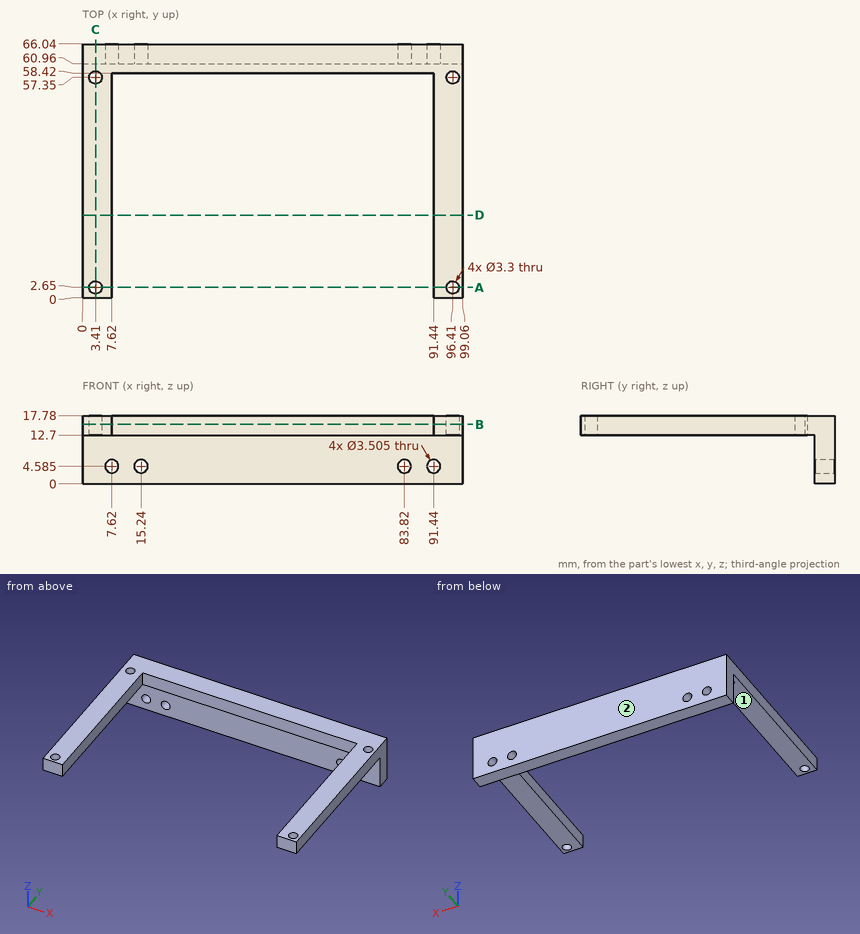
Part print with two shaded views. Sizes in mm from the minimum x, y, z corner. A direction names the side the tool comes from. Round coordinates to 2 decimals unless told otherwise and drop trailing zeros. Write each loop counter-clockwise with the first axis right and the second up, starting at its lowest first coordinate (ties: lowest second). Pieces come first, ordered by that corner, then holes. Notation, with made-up numbers: (38.5, -26) - (94.5, -26) arc R14 cw to (94.5, -22) - close; hole circle Ø7 at (65, 81). An arc over 180 degrees is marked (long way). Use CSV: the item, a comma, the result in double quotes.
Item 1: Slice it at D-D, the plane y = 21.5. Write the cut outline in (x, z), then the cut area to 3 significant figures.
Results list:
outline,"(0, 12.7) - (7.62, 12.7) - (7.62, 17.78) - (0, 17.78) - close; (91.44, 12.7) - (99.06, 12.7) - (99.06, 17.78) - (91.44, 17.78) - close"
area,"77.4 mm²"
Item 2: Flat gauge pins, fed straight in: P1, Ø2.5, axis at x = 3.41, y = 57.35, coming from the +Z side; P2, Ø1.5, axis at x = 43, z = 15, coming from the -Y side; P3, Ø6.5, axis at x = 47, z = 6.5, coming from the -Y side. Where does each tip first touch, or does it go through?
Results list:
P1,"passes through"
P2,"stops at y = 58.42"
P3,"stops at y = 60.96"
Item 3: Slice it at B-B, the plane z = 15.5. Write the cut outline in (x, y).
Results list:
outline,"(0, 0) - (7.62, 0) - (7.62, 58.42) - (91.44, 58.42) - (91.44, 0) - (99.06, 0) - (99.06, 66.04) - (0, 66.04) - close; hole circle Ø3.3 at (3.41, 2.65); hole circle Ø3.3 at (3.41, 57.35); hole circle Ø3.3 at (96.41, 2.65); hole circle Ø3.3 at (96.41, 57.35)"
Item 4: Wall check: L1, parallel to X at y = 23, z = 15; L2, parallel to Y at x = 36, z = 12; L3, parallel to Z at x = 91.44, y = 62.65. Give the ranges that are in metal, low to high.
Results list:
L1,"x = 0 to 7.62, 91.44 to 99.06"
L2,"y = 60.96 to 66.04"
L3,"z = 0 to 2.83, 6.34 to 17.78"
Item 5: Tool access for the marked faces 1 and 2: list every direction of +Z, -Z, +X, -X, +Y, -Y with a clear straight run to the whole face (end or side of a thin tool).
Results list:
face 1,"-Z, +X, -X, -Y"
face 2,"+Z, -Z, +X, -X, +Y"
Item 6: Slice it at C-C, the plane x = 3.41. Write the cut outline in (y, z).
Results list:
outline,"(0, 12.7) - (1, 12.7) - (1, 17.78) - (0, 17.78) - close; (4.3, 12.7) - (55.7, 12.7) - (55.7, 17.78) - (4.3, 17.78) - close; (59, 12.7) - (60.96, 12.7) - (60.96, 0) - (66.04, 0) - (66.04, 17.78) - (59, 17.78) - close"
Item 7: Slice it at A-A, the plane y = 2.65. Write the cut outline in (x, z).
Results list:
outline,"(0, 12.7) - (1.76, 12.7) - (1.76, 17.78) - (0, 17.78) - close; (5.06, 12.7) - (7.62, 12.7) - (7.62, 17.78) - (5.06, 17.78) - close; (91.44, 12.7) - (94.76, 12.7) - (94.76, 17.78) - (91.44, 17.78) - close; (98.06, 12.7) - (99.06, 12.7) - (99.06, 17.78) - (98.06, 17.78) - close"
